Part model, mm, in its own coordinate system. Face numbers are marked on the shaded views. A direction names the side the tool comes from. Coordinates: 2 decimals unless noted, no trailing zeros. Loops run counter-clockwise (first coordinate to the right, second up) from the corner with the lowest first, then second, coordinate; pieces in that order, holes last.
```python
from build123d import *

# Parameters (mm, degrees)
SKETCH1_W           = 39.5
SKETCH1_H           = 27.5
SKETCH1_R           = 2.5
BOSS_EXTRUDE1_DEPTH = 3
SKETCH3_W           = 3
SKETCH3_H           = 27.5
BOSS_EXTRUDE2_DEPTH = 36.5
SKETCH4_R           = 2.5
CUT_EXTRUDE1_DEPTH  = 36.5
FILLET1_R           = 2


with BuildPart() as part:
    # Sketch1 → Boss-Extrude1 (new body)
    with BuildSketch(Plane.XY):
        with Locations((-17.382808989, -12.897191011)):
            Rectangle(SKETCH1_W, SKETCH1_H)
        with Locations((-24.632808989, -12.897191011)):
            Circle(SKETCH1_R, mode=Mode.SUBTRACT)
        with Locations((-7.132808989, -12.897191011)):
            Circle(SKETCH1_R, mode=Mode.SUBTRACT)
    extrude(amount=BOSS_EXTRUDE1_DEPTH)

    # Sketch3 → Boss-Extrude2 (add)
    with BuildSketch(Plane(origin=(0, 0, 0), x_dir=(-1, 0, 0), z_dir=(0, 0, -1))):
        with Locations((35.632808989, -12.897191011)):
            Rectangle(SKETCH3_W, SKETCH3_H)
    extrude(amount=BOSS_EXTRUDE2_DEPTH)

    # Sketch4 → Cut-Extrude1 (cut)
    with BuildSketch(Plane(origin=(-34.132808989, 0, 0), x_dir=(0, 0, -1), z_dir=(1, 0, 0))):
        with Locations((9.5, -12.897191011)):
            Circle(SKETCH4_R)
        with Locations((27, -12.897191011)):
            Circle(SKETCH4_R)
    extrude(amount=-CUT_EXTRUDE1_DEPTH, mode=Mode.SUBTRACT)

    # Fillet1
    fillet1_edges = [part.edges().sort_by_distance(p)[0] for p in [
        (-37.132808989, -12.897191011, 3),
    ]]
    fillet(fillet1_edges, radius=FILLET1_R)


solid = part.part
```
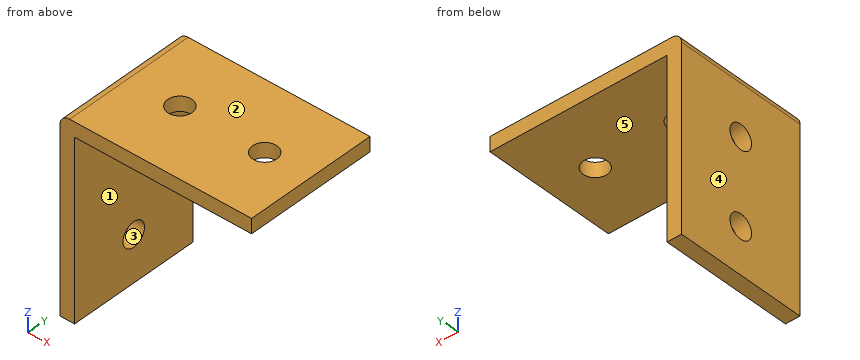
Q1. Saw through at B-B (y = -9.75). List the corners of the cut face in (x, z).
Q2. Saw through at A-A (z = -27). List the corners of the cut face in (x, y).
Q3. Saw through at C-C (x = -24). List the corners of the cut face in (y, z).
Q4. Drop flat-ended pins along their axis: P1, Ø6, axis at x = -32.5, z = -32, coming from the -Y side; P2, Ø6, axis at y = -2.5, z = -20.5, coming from the +X side; P3, Ø5, axis at x = -21.5, y = -4.5, coming from the -Z side. Give the stop position or say it passes through.
Q5. Saw through at D-D (x = -16.5). List the corners of the cut face in (y, z).
Q6. Tool access for the marked faces 4 and 5: list every direction of +Z, -Z, +X, -X, +Y, -Y with a clear straight run to the whole face (end or side of a thin tool).
Q7. Mould opens along Z. For the marked faces 1, 2 and 3 say: released by +Z, released by -Z, zero draft, split by the parting line, or undercut.
Q8. Probe line 1 (Y direction, x = -34.8, z = -27); line 2 (Z direction, x = -35, y = -13.5); line 3 (X direction, y = -16, z = -24.5). List the from-to ranges inside material, lowest first.
Checked values:
1. outline: (-37.13, -36.5) - (-34.13, -36.5) - (-34.13, 0) - (2.37, 0) - (2.37, 3) - (-35.13, 3) arc R2 ccw to (-37.13, 1) - close
2. outline: (-37.13, -26.65) - (-34.13, -26.65) - (-34.13, -15.4) - (-37.13, -15.4) - close; (-37.13, -10.4) - (-34.13, -10.4) - (-34.13, 0.85) - (-37.13, 0.85) - close
3. outline: (-26.65, 0) - (-15.32, 0) - (-15.32, 3) - (-26.65, 3) - close; (-10.48, 0) - (0.85, 0) - (0.85, 3) - (-10.48, 3) - close
4. P1: stops at y = -26.65
4. P2: stops at x = -34.13
4. P3: stops at z = 0
5. outline: (-26.65, 0) - (0.85, 0) - (0.85, 3) - (-26.65, 3) - close
6. face 4: +Z, -Z, -X, +Y, -Y
6. face 5: -Z, +X, +Y, -Y
7. face 1: zero draft
7. face 2: released by +Z
7. face 3: undercut
8. line 1: y = -26.65 to -15.4, -10.4 to 0.85
8. line 2: z = -36.5 to -29.43, -24.57 to -11.93, -7.07 to 3
8. line 3: x = -37.13 to -34.13
